Verification items for the finished model (mm, model axes). A direction names the side the tool comes from. Coordinates: 2 decimals unless noted, no trailing zeros. Order: outer loops, then holes, each group sorted by start corner. A loop starts at its lowest first (then second) coordinate and runs counter-clockwise, first axis right, second up. Notation, with made-up numbers: M -17.75,-35.5 L 17.25,-35.5 A28 ccw 17.25,0.5 Z; hole C 32,88.25 d10. An arc over 180 degrees is marked long. Return JSON: item names as keys, results as strings. Group by question number.
Q1. Section check A-A, the plane y = 2.75. Enter the section's corners in (x, z).
Q2. Go/stop test with flat-tipped pins: pin 1 Ø6 at (x, y) = (-30, 1) entering from +Z; pin 2 Ø1.5 at (x, z) = (-93, -9) entering from +Y; pin 3 Ø1.5 at (x, y) = (-104.5, 3) entering from -Z. Record where each tip stops, or that it passes through.
Q3. Thickness scan on probe 1 along Y at (x, z) = (0, -7.5); probe 2 along Z at (x, y) = (-109, 0.25). Record the ranges inside material, lowest first.
Q4. Access from +Z, -Z, +X, -X, +Y, -Y to the whole of each face (thin tool, end or side, straight path). Record for faces 3 (the face through (-0.75, -5.7, -7.05)), 4 (the face through (-108.67, 2.3, -16.04)).
Q5. Section check C-C, the plane y = -3.5. Enter the section's corners in (x, z), then the cut area to 3 significant figures.
Q6. Mould release check, pull along Y, two halves, no side actions. Record for faces 1 (the face through (-53.542, -4.055, -12.164)), 2 (the face through (-53.346, -0.253, -10.856)): pulls with the +Y half, pulls with the -Y half, needs draft (parallel to the pull), parting line crosses it, or undercut.
Q7. Section check B-B, the plane z = -10.5. Count the separate pieces of the cut face and the enclosed holes in it, then the cut area to 3 significant figures.
from build123d import *

# Parameters (mm, degrees)
F0_R   = 6
F0_R_2 = 5.75


with BuildPart() as f2:
    # F2: sweep along a path in F1
    with BuildLine(Plane.XZ) as f2_path:
        Line((-6, 0), (-6, -13.9078725958))
        ThreePointArc((-6, -13.9078725958), (-7.0345199545, -16.1743430215), (-9.4245921271, -16.8776741928))
        Line((-9.4245921271, -16.8776741928), (-96, -4.5))
        Line((-96, -4.5), (-121, -4.5))
    # F0 (on Top) → F2 (sweep)
    with BuildSketch(Plane.XY):
        Circle(F0_R)
        Circle(F0_R_2, mode=Mode.SUBTRACT)
    sweep(path=f2_path.line, transition=Transition.RIGHT)


solid = f2.part
Numbers:
{
 "1": {"outline": "M -121,-15.83 L -96.81,-15.83 L -11.03,-28.1 A14.33 ccw 5.33,-13.91 L 5.33,0 L 5.05,0 L 5.05,-13.91 A14.05 cw -10.99,-27.82 L -96.79,-15.55 L -121,-15.55 Z; M -121,-5.45 L -96.07,-5.45 L -9.56,-17.82 A3.95 ccw -5.05,-13.91 L -5.05,0 L -5.33,0 L -5.33,-13.91 A3.67 cw -9.52,-17.54 L -96.05,-5.17 L -121,-5.17 Z"},
 "2": {"pin 1": "stops at z = -13.53", "pin 2": "stops at y = 5.87", "pin 3": "stops at z = -16.06"},
 "3": {"probe 1": "y = -6 to -5.75, 5.75 to 6", "probe 2": "z = -16.49 to -16.24, -4.76 to -4.51"},
 "4": {"face 3": "+Z", "face 4": "-X"},
 "5": {"outline": "M -121,-15.37 L -96.77,-15.37 L -10.96,-27.64 A13.87 ccw 4.87,-13.91 L 4.87,0 L 4.56,0 L 4.56,-13.91 A13.56 cw -10.92,-27.33 L -96.75,-15.06 L -121,-15.06 Z; M -121,-5.94 L -96.1,-5.94 L -9.63,-18.3 A4.44 ccw -4.56,-13.91 L -4.56,0 L -4.87,0 L -4.87,-13.91 A4.13 cw -9.58,-17.99 L -96.08,-5.63 L -121,-5.63 Z", "area": "87.7 mm2"},
 "6": {"face 1": "parting line crosses it", "face 2": "undercut"},
 "7": {"separate pieces": "2", "enclosed holes": "1", "area": "54.1 mm2"}
}
